Design review of the part shown in the three views and the two pictorial views. Dimensions are in mm from the part's minimum x, y and z. Give positions to 0.01 mm unless a question says otherwise; leave off trailing zeros. Loops run counter-clockwise (first coordinate to the right, second up) from the corner with the lowest first, then second, coordinate; pieces in that order, holes last. Notation, with made-up numbers: (40, 39.25) -> (75, 39.25) arc R22 cw to (75, 53.25) -> close; hole circle Ø2 at (-33, 46.25). An arc over 180 degrees is marked (long way). One line per question, with ' | ' between items. Start each with the question number.
(1) Consider section D-D (z = 60). Write out the cut boundary in (x, y).
(2) Insertion check: P1, Ø1.1, axis at y = 0.5, z = 26.5, coming from the -X side; P2, Ø2.5, axis at x = 74.5, z = 29.5, coming from the +Y side; P3, Ø12, axis at x = 13, z = 30.5, coming from the -Y side; P4, Ø2, axis at x = 50.5, y = 1.5, coming from the -Z side. Each pin has a flat end and moves straight along its axis. Give the tip position at first contact, or say it passes through.
(3) Consider section B-B (z = 51). Write out the cut boundary in (x, y), and give its area (3 significant figures).
(4) Consider section A-A (x = 75). Write out the cut boundary in (y, z), and give its area (3 significant figures).
(5) Consider section C-C (y = 2.6). Write out the cut boundary in (x, z).
(6) Wall thickness on probe 1 along X at (y, z) = (2.35, 3); probe 2 along X at (y, z) = (1.7, 4); probe 3 along Z at (x, y) = (18, 0.6): over which ranges is each line inside the solid? List them lowest first.
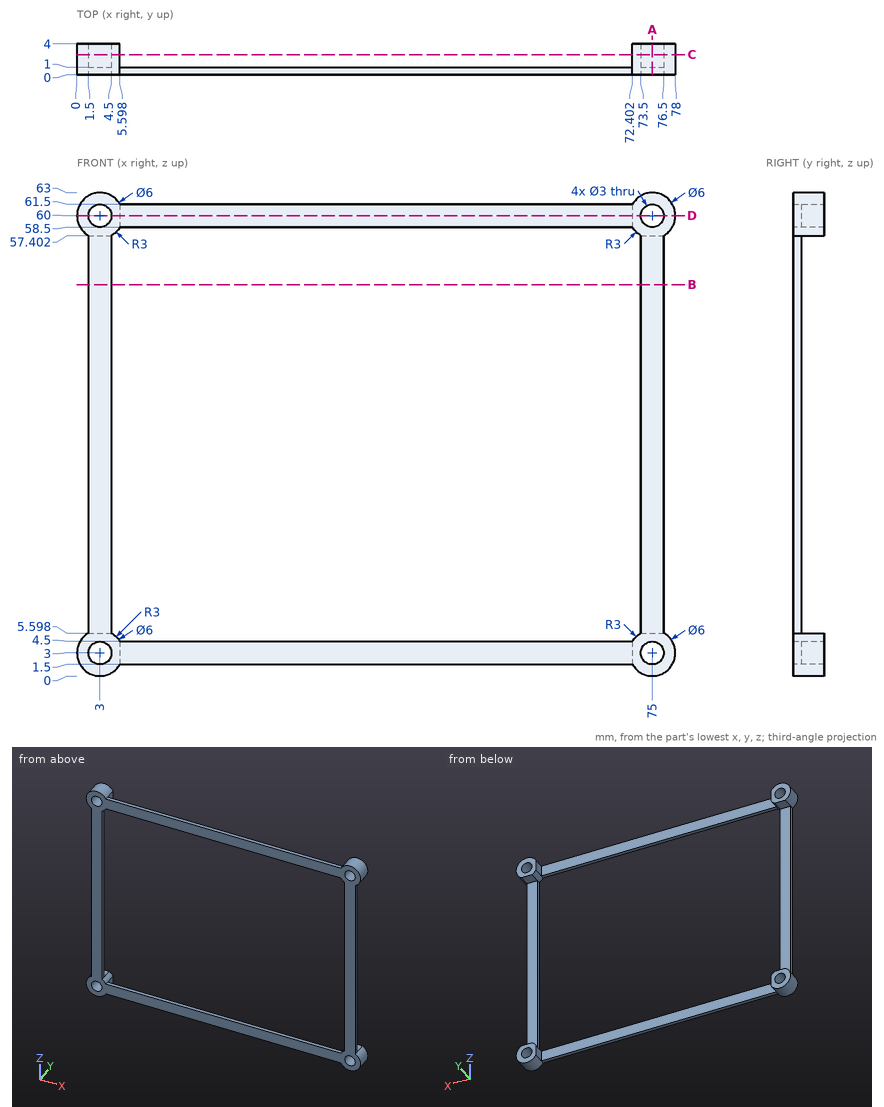
A:
1) outline: (0, 0) -> (1.5, 0) -> (1.5, 4) -> (0, 4) -> close; (4.5, 0) -> (73.5, 0) -> (73.5, 4) -> (72.4, 4) -> (72.4, 1) -> (5.6, 1) -> (5.6, 4) -> (4.5, 4) -> close; (76.5, 0) -> (78, 0) -> (78, 4) -> (76.5, 4) -> close
2) P1: stops at x = 1.5 | P2: stops at y = 1 | P3: passes through | P4: stops at z = 1.5
3) outline: (1.5, 0) -> (4.5, 0) -> (4.5, 1) -> (1.5, 1) -> close; (73.5, 0) -> (76.5, 0) -> (76.5, 1) -> (73.5, 1) -> close | area: 6.00 mm^2
4) outline: (0, 0) -> (4, 0) -> (4, 1.5) -> (0, 1.5) -> close; (0, 4.5) -> (4, 4.5) -> (4, 5.6) -> (1, 5.6) -> (1, 57.4) -> (4, 57.4) -> (4, 58.5) -> (0, 58.5) -> close; (0, 61.5) -> (4, 61.5) -> (4, 63) -> (0, 63) -> close | area: 72.6 mm^2
5) outline: (1.5, 5.6) arc R3 ccw (long way) to (5.6, 1.5) -> (5.6, 4.5) arc R3 ccw to (4.5, 5.6) -> close; (1.5, 57.4) -> (4.5, 57.4) arc R3 ccw to (5.6, 58.5) -> (5.6, 61.5) arc R3 ccw (long way) to start; (72.4, 1.5) arc R3 ccw (long way) to (76.5, 5.6) -> (73.5, 5.6) arc R3 ccw to (72.4, 4.5) -> close; (72.4, 58.5) arc R3 ccw to (73.5, 57.4) -> (76.5, 57.4) arc R3 ccw (long way) to (72.4, 61.5) -> close; hole circle Ø3 at (3, 3); hole circle Ø3 at (3, 60); hole circle Ø3 at (75, 3); hole circle Ø3 at (75, 60)
6) probe 1: x = 0 to 1.5, 4.5 to 5.6, 72.4 to 73.5, 76.5 to 78 | probe 2: x = 0.17 to 1.88, 4.12 to 5.6, 72.4 to 73.88, 76.12 to 77.83 | probe 3: z = 1.5 to 4.5, 58.5 to 61.5
